```python
from build123d import *

# Parameters (mm, degrees)
BOSS_EXTRUDE1_DEPTH = 0.6
SKETCH2_R           = 1.1
CUT_EXTRUDE1_DEPTH  = 22.075696904
SKETCH3_W           = 12.15
SKETCH3_H           = 10.57
SKETCH3_W_2         = 2
SKETCH3_H_2         = 7
BOSS_EXTRUDE2_DEPTH = 1.8
SKETCH4_W           = 4.75
SKETCH4_H           = 7.9
BOSS_EXTRUDE3_DEPTH = 8.75
FILLET1_R           = 1


with BuildPart() as part:
    # Sketch1 → Boss-Extrude1 (new body)
    with BuildSketch(Plane(origin=(0, 0, 0), x_dir=(1, 0, 0), z_dir=(0, 1, 0))):
        with BuildLine():
            Line((6.175, 10.05), (-6.175, 10.05))
            Line((-6.175, 10.05), (-6.175, 13))
            Line((-6.175, 13), (-11.675, 13))
            Line((-11.675, 13), (-11.675, 2.960451824))
            ThreePointArc((-11.675, 2.960451824), (-12.549347485, -1.851203428), (-8.075, -3.82521568))
            Line((-8.075, -3.82521568), (-8.075, -16.57))
            Line((-8.075, -16.57), (8.075, -16.57))
            Line((8.075, -16.57), (8.075, -3.82521568))
            ThreePointArc((8.075, -3.82521568), (12.549347485, -1.851203428), (11.675, 2.960451824))
            Line((11.675, 2.960451824), (11.675, 13))
            Line((11.675, 13), (6.175, 13))
            Line((6.175, 13), (6.175, 10.05))
        make_face()
    extrude(amount=BOSS_EXTRUDE1_DEPTH)

    # Sketch2 → Cut-Extrude1 (cut, through all)
    with BuildSketch(Plane(origin=(0, 0.6, 0), x_dir=(1, 0, 0), z_dir=(0, 1, 0))):
        with Locations(Location((-9.1, 0, 0), (0, 0, 270))):
            Circle(SKETCH2_R)
        with Locations(Location((9.1, 0, 0), (0, 0, 90))):
            Circle(SKETCH2_R)
    extrude(amount=-CUT_EXTRUDE1_DEPTH, mode=Mode.SUBTRACT)

    # Sketch3 → Boss-Extrude2 (add)
    with BuildSketch(Plane.XZ):
        with Locations((0, 10.285)):
            Rectangle(SKETCH3_W, SKETCH3_H)
        with Locations((-9.675, -8.5)):
            Rectangle(SKETCH3_W_2, SKETCH3_H_2)
        with Locations((9.675, -8.5)):
            Rectangle(SKETCH3_W_2, SKETCH3_H_2)
    extrude(amount=BOSS_EXTRUDE2_DEPTH)

    # Sketch4 → Boss-Extrude3 (add)
    with BuildSketch(Plane(origin=(0, 0.6, 0), x_dir=(1, 0, 0), z_dir=(0, 1, 0))):
        with Locations((-9.05, 8.55)):
            Rectangle(SKETCH4_W, SKETCH4_H)
        with Locations((9.05, 8.55)):
            Rectangle(SKETCH4_W, SKETCH4_H)
    extrude(amount=BOSS_EXTRUDE3_DEPTH)

    # Fillet1
    fillet1_edges = [part.edges().sort_by_distance(p)[0] for p in [
        (-6.175, 0.3, -10.05),
        (6.175, 0.3, -10.05),
        (8.075, 0.3, 3.82521568),
        (-8.075, 0.3, 3.82521568),
    ]]
    fillet(fillet1_edges, radius=FILLET1_R)


solid = part.part
```
Geometry: final body of the model. Coordinates: model frame, mm. A direction names the side the tool comes from. Give positions to 0.01 mm unless a question says otherwise; leave off trailing zeros. Order: outer loops, then holes, each group sorted by start corner. A loop starts at its lowest first (then second) coordinate and runs counter-clockwise, first axis right, second up. Notation, with made-up numbers: (-20, 49) -> (20, 49) arc R27 ccw to (20, 86) -> close; hole circle Ø4 at (76, 31.5). An arc over 180 degrees is marked (long way). Write each question's results on one line, items separated by ' | '. Start each with the question number.
1) Draft query along X for faces 1 (the flat face through (0, 0, -2)), 2 (the cylindrical face through (8.37, 0.3, 4.24)), 3 (the flat face through (10, -1.8, -8)). Return one class per face: pulls with the +X half, pulls with the -X half, needs draft (parallel to the pull), parting line crosses it, or undercut.
2) Line query: line 1 (X direction, y = 0.45, z = 0); line 2 (Z direction, x = 9.1, y = 0.3); line 3 (Z direction, x = 8, y = 4.5). Output: solid intervals per line, ascending. Write a range as from..to.
3) First-contact query: pin 1 (1.5 mm diameter, centred on y = 0, z = -7.5, fed in from -X) (3 decimals); pin 2 (2 mm diameter, centred on x = 6, z = 5.5, fed in from +Y); pin 3 (0.5 mm diameter, centred on x = 9.5, y = -1, fed in from -Z). Flat tips, straight axial feed; report the tip coordinate or a pass-through.
4) Section B-B (y = 5.5). Return loops of the section in (x, z) (3 decimals), then the cut area to 4 significant figures.
5) Section C-C (x = -7.5). Return loops of the section in (y, z), then the cut area to 3 significant figures.
6) Section D-D (z = 9.5). Return loops of the section in (x, y) (3 decimals).
7) Section A-A (z = 0). Return loops of the section in (x, y).
8) Set-up query: faces 4 (the flat face through (6.075, -1, 10)), 5 (the flat face through (0, -1, 5)), 6 (the flat face through (0, -1, 15.57)), 7 (the flat face through (-9, 5, -12.5)). Return all of +Z, -Z, +X, -X, +Y, -Y with unobstructed straight access to the full face (end or side cutting, diameter ignored); none if empty.
Calculated:
1) face 1: undercut | face 2: pulls with the +X half | face 3: needs draft
2) line 1: -13.01..-10.2, -8..8, 10.2..13.01 | line 2: -13..-1.1, 1.1..3.95 | line 3: -12.5..-4.6
3) pin 1: x = -11.675 | pin 2: y = 0.6 | pin 3: z = -12
4) outline: (-11.425, -12.5) -> (-6.675, -12.5) -> (-6.675, -4.6) -> (-11.425, -4.6) -> close; (6.675, -12.5) -> (11.425, -12.5) -> (11.425, -4.6) -> (6.675, -4.6) -> close | area: 75.05 mm2
5) outline: (0, -13) -> (0.6, -13) -> (0.6, -12.5) -> (9.35, -12.5) -> (9.35, -4.6) -> (0.6, -4.6) -> (0.6, 16.57) -> (0, 16.57) -> close | area: 86.9 mm2
6) outline: (-8.075, 0) -> (-6.075, 0) -> (-6.075, -1.8) -> (6.075, -1.8) -> (6.075, 0) -> (8.075, 0) -> (8.075, 0.6) -> (-8.075, 0.6) -> close
7) outline: (-13.01, 0) -> (-10.2, 0) -> (-10.2, 0.6) -> (-13.01, 0.6) -> close; (-8, 0) -> (8, 0) -> (8, 0.6) -> (-8, 0.6) -> close; (10.2, 0) -> (13.01, 0) -> (13.01, 0.6) -> (10.2, 0.6) -> close
8) face 4: +Z, -Z, +X, -Y | face 5: -Z, +X, -X, -Y | face 6: +Z, +X, -X, -Y | face 7: -Z, +X, -X, +Y
